Read the model definition and answer for the solid it produces. Units are mm, in the model's axes. A direction names the side the tool comes from. Coordinates: 2 decimals unless noted, no trailing zeros. Write each loop counter-clockwise with the first axis right and the second up, starting at its lowest first coordinate (ties: lowest second). Pieces come first, ordered by that corner, then holes. Notation, with made-up numbers: (3, 74) - (61, 74) arc R14 cw to (61, 100) - close; hole circle Ø2 at (0.25, 32.25). An arc over 180 degrees is marked (long way). Use a Markdown table: item, result.
from build123d import *

# Parameters (mm, degrees)
SKETCH_1_W                   = 1300
SKETCH_1_H                   = 272
SM_BASE_FLANGE_1_DEPTH       = 0.8
SM_START                     = -650
SM_EDGE_FLANGE_1_DEPTH       = 1300
SM_START_2                   = -490
SM_EDGE_FLANGE_1_2_OUTLINE_W = 0.8
SM_EDGE_FLANGE_1_2_OUTLINE_H = 24.2
SM_EDGE_FLANGE_1_2_DEPTH     = 980
SM_EDGE_FLANGE_1_3_OUTLINE_W = 0.8
SM_EDGE_FLANGE_1_3_OUTLINE_H = 4.2
SM_EDGE_FLANGE_1_3_DEPTH     = 1300
SKETCH_11_R                  = 3
CUT_EXTRUDE_1_DEPTH          = 706.059571951
SM_START_3                   = -131.8
SM_EDGE_FLANGE_2_DEPTH       = 263.6
SM_EDGE_FLANGE_2_2_DEPTH     = 0.8
SM_START_4                   = 131
SM_EDGE_FLANGE_2_3_DEPTH     = 0.8
SM_START_5                   = -48
SM_EDGE_FLANGE_2_4_OUTLINE_W = 0.8
SM_EDGE_FLANGE_2_4_OUTLINE_H = 24.2
SM_EDGE_FLANGE_2_4_DEPTH     = 154
SM_START_6                   = -131
SM_EDGE_FLANGE_2_5_OUTLINE_W = 0.8
SM_EDGE_FLANGE_2_5_OUTLINE_H = 4.2
SM_EDGE_FLANGE_2_5_DEPTH     = 262
SKETCH_15_R                  = 3
CUT_EXTRUDE_2_DEPTH          = 1308.33354581


# Read off the part's stored shape, not the designer's step: 边线-法兰1, 边线-法兰2
# Sheet-metal steps are written as plain solids
with BuildPart() as part:
    # Sketch 1 → 基体-法兰1 (new body)
    with BuildSketch(Plane.XY):
        Rectangle(SKETCH_1_W, SKETCH_1_H)
    extrude(amount=-SM_BASE_FLANGE_1_DEPTH)

    # 边线-法兰1 outline → 边线-法兰1 (cut)
    with BuildSketch(Plane.YZ.offset(SM_START)):
        with BuildLine():
            Line((136, 0), (135.2, 0))
            ThreePointArc((135.2, 0), (135.765685425, -0.234314575), (136, -0.8))
            Line((136, -0.8), (136, 0))
        make_face()
    sm_edge_flange_1 = extrude(amount=SM_EDGE_FLANGE_1_DEPTH, mode=Mode.SUBTRACT)

    # Sm Edge Flange 1 2 outline → Sm Edge Flange 1 2 (add)
    with BuildSketch(Plane.YZ.offset(SM_START_2)):
        with Locations((135.6, -12.9)):
            Rectangle(SM_EDGE_FLANGE_1_2_OUTLINE_W, SM_EDGE_FLANGE_1_2_OUTLINE_H)
    sm_edge_flange_1_2 = extrude(amount=SM_EDGE_FLANGE_1_2_DEPTH)

    # Sm Edge Flange 1 3 outline → Sm Edge Flange 1 3 (add)
    with BuildSketch(Plane.YZ.offset(SM_START)):
        with Locations((135.6, -2.9)):
            Rectangle(SM_EDGE_FLANGE_1_3_OUTLINE_W, SM_EDGE_FLANGE_1_3_OUTLINE_H)
    sm_edge_flange_1_3 = extrude(amount=SM_EDGE_FLANGE_1_3_DEPTH)

    # 镜向1: 边线-法兰1, Sm Edge Flange 1 2, Sm Edge Flange 1 3 across plane
    add(sm_edge_flange_1.mirror(Plane.ZX), mode=Mode.SUBTRACT)
    add(sm_edge_flange_1_2.mirror(Plane.ZX))
    add(sm_edge_flange_1_3.mirror(Plane.ZX))

    # 草图11 → 切除-拉伸1 (cut, through all)
    with BuildSketch(Plane(origin=(0, 136, 0), x_dir=(1, 0, 0), z_dir=(0, 1, 0))):
        with Locations(Location((0, 15, 0), (0, 0, 270))):
            Circle(SKETCH_11_R)
        with Locations(Location((230, 15, 0), (0, 0, 270))):
            Circle(SKETCH_11_R)
        with Locations(Location((460, 15, 0), (0, 0, 270))):
            Circle(SKETCH_11_R)
        with Locations(Location((-230, 15, 0), (0, 0, 270))):
            Circle(SKETCH_11_R)
        with Locations(Location((-460, 15, 0), (0, 0, 270))):
            Circle(SKETCH_11_R)
    extrude(amount=-CUT_EXTRUDE_1_DEPTH, mode=Mode.SUBTRACT)

    # 边线-法兰2 outline → 边线-法兰2 (cut)
    with BuildSketch(Plane(origin=(0, 0, 0), x_dir=(1, 0, 0), z_dir=(0, 1, 0)).offset(SM_START_3)):
        with BuildLine():
            ThreePointArc((-649.2, 0), (-649.765685425, 0.234314575), (-650, 0.8))
            Line((-650, 0.8), (-650, 0))
            Line((-650, 0), (-649.2, 0))
        make_face()
    sm_edge_flange_2 = extrude(amount=SM_EDGE_FLANGE_2_DEPTH, mode=Mode.SUBTRACT)

    # Sm Edge Flange 2 2 outline → Sm Edge Flange 2 2 (cut)
    with BuildSketch(Plane(origin=(0, 0, 0), x_dir=(1, 0, 0), z_dir=(0, 1, 0)).offset(SM_START_3)):
        with BuildLine():
            Line((-648.4, 0.8), (-650, 0.8))
            ThreePointArc((-650, 0.8), (-649.765685425, 0.234314575), (-649.2, 0))
            Line((-649.2, 0), (-648.4, 0))
            Line((-648.4, 0), (-648.4, 0.8))
        make_face()
    sm_edge_flange_2_2 = extrude(amount=SM_EDGE_FLANGE_2_2_DEPTH, mode=Mode.SUBTRACT)

    # Sm Edge Flange 2 3 outline → Sm Edge Flange 2 3 (cut)
    with BuildSketch(Plane(origin=(0, 0, 0), x_dir=(1, 0, 0), z_dir=(0, 1, 0)).offset(SM_START_4)):
        with BuildLine():
            Line((-648.4, 0.8), (-650, 0.8))
            ThreePointArc((-650, 0.8), (-649.765685425, 0.234314575), (-649.2, 0))
            Line((-649.2, 0), (-648.4, 0))
            Line((-648.4, 0), (-648.4, 0.8))
        make_face()
    sm_edge_flange_2_3 = extrude(amount=SM_EDGE_FLANGE_2_3_DEPTH, mode=Mode.SUBTRACT)

    # Sm Edge Flange 2 4 outline → Sm Edge Flange 2 4 (add)
    with BuildSketch(Plane(origin=(0, 0, 0), x_dir=(1, 0, 0), z_dir=(0, 1, 0)).offset(SM_START_5)):
        with Locations((-649.6, 12.9)):
            Rectangle(SM_EDGE_FLANGE_2_4_OUTLINE_W, SM_EDGE_FLANGE_2_4_OUTLINE_H)
    sm_edge_flange_2_4 = extrude(amount=SM_EDGE_FLANGE_2_4_DEPTH)

    # Sm Edge Flange 2 5 outline → Sm Edge Flange 2 5 (add)
    with BuildSketch(Plane(origin=(0, 0, 0), x_dir=(1, 0, 0), z_dir=(0, 1, 0)).offset(SM_START_6)):
        with Locations((-649.6, 2.9)):
            Rectangle(SM_EDGE_FLANGE_2_5_OUTLINE_W, SM_EDGE_FLANGE_2_5_OUTLINE_H)
    sm_edge_flange_2_5 = extrude(amount=SM_EDGE_FLANGE_2_5_DEPTH)

    # 镜向2: 边线-法兰2, Sm Edge Flange 2 2, Sm Edge Flange 2 3, Sm Edge Flange 2 4, Sm Edge Flange 2 5 across plane
    add(sm_edge_flange_2.mirror(Plane(origin=(0, 0, 0), x_dir=(0, 0, 1), z_dir=(1, 0, 0))), mode=Mode.SUBTRACT)
    add(sm_edge_flange_2_2.mirror(Plane(origin=(0, 0, 0), x_dir=(0, 0, 1), z_dir=(1, 0, 0))), mode=Mode.SUBTRACT)
    add(sm_edge_flange_2_3.mirror(Plane(origin=(0, 0, 0), x_dir=(0, 0, 1), z_dir=(1, 0, 0))), mode=Mode.SUBTRACT)
    add(sm_edge_flange_2_4.mirror(Plane(origin=(0, 0, 0), x_dir=(0, 0, 1), z_dir=(1, 0, 0))))
    add(sm_edge_flange_2_5.mirror(Plane(origin=(0, 0, 0), x_dir=(0, 0, 1), z_dir=(1, 0, 0))))

    # 草图15 → 切除-拉伸2 (cut, through all)
    with BuildSketch(Plane.ZY.offset(650)):
        with Locations((-15, 0)):
            Circle(SKETCH_15_R)
    extrude(amount=-CUT_EXTRUDE_2_DEPTH, mode=Mode.SUBTRACT)


solid = part.part
(1) A cutting plane is placed at B-B, the plane x = -261. Write down the section's boundary in (y, z), and give its area (3 significant figures).
Report:
| item | result |
|---|---|
| outline | (-136, -25) - (-135.2, -25) - (-135.2, -0.8) - (135.2, -0.8) - (135.2, -25) - (136, -25) - (136, -0.8) arc R0.8 ccw to (135.2, 0) - (-135.2, 0) arc R0.8 ccw to (-136, -0.8) - close |
| area | 256 mm² |
(2) Each of these flat-tipped pins is pushed along its axis until it touches: P1, Ø3, axis at x = -394.5, y = 31, coming from the +Z side; P2, Ø0.9, axis at x = 649.5, y = 114.5, coming from the -Z side; P3, Ø6, axis at x = -302.5, y = 43.5, coming from the -Z side; P4, Ø0.6, axis at y = 135.5, z = -14, coming from the -X side. Where does it stop, or does it pass through?
Report:
| item | result |
|---|---|
| P1 | stops at z = 0 |
| P2 | stops at z = -5 |
| P3 | stops at z = -0.8 |
| P4 | stops at x = -490 |
(3) Straight lines are drawn through the part: L1, parallel to X at y = -135.35, z = -15; L2, parallel to Z at x = 230, y = 135.4; L3, parallel to Y at x = -21, z = -17.5. For each, find the intervals that lie inside material, in ascending order.
Report:
| item | result |
|---|---|
| L1 | x = -490 to -463, -457 to -233, -227 to -3, 3 to 227, 233 to 457, 463 to 490 |
| L2 | z = -25 to -18, -12 to -0.03 |
| L3 | y = -136 to -135.2, 135.2 to 136 |
(4) The mould has two halves that part along Y. Classify faces 1 (the flat face through (-9, 2, 0)), 2 (the flat face through (-9, -136, -13)), 3 (the flat face through (-9, 2, -0.8)): pulls with the +Y half, pulls with the -Y half, needs draft (parallel to the pull), parting line crosses it, or undercut.
Report:
| item | result |
|---|---|
| face 1 | needs draft |
| face 2 | pulls with the -Y half |
| face 3 | undercut |
(5) A cutting plane is placed at A-A, the plane y = -76. Write down the section's boundary in (x, z), and give its area (3 significant figures).
Report:
| item | result |
|---|---|
| outline | (-650, -5) - (-649.2, -5) - (-649.2, -0.8) - (649.2, -0.8) - (649.2, -5) - (650, -5) - (650, -0.8) arc R0.8 ccw to (649.2, 0) - (-649.2, 0) arc R0.8 ccw to (-650, -0.8) - close |
| area | 1,050 mm² |
(6) For faces 4 (the flat face through (-9, 136, -13)), 5 (the flat face through (-9, -135.2, -13)), 6 (the flat face through (649.2, 27, -10)), determine the directions among +Z, -Z, +X, -X, +Y, -Y from which every point of the face is accessible in a straight line to the end or side of a thin tool.
Report:
| item | result |
|---|---|
| face 4 | +Z, -Z, +X, -X, +Y |
| face 5 | -Z, +X, -X |
| face 6 | -Z |
